Verification items for the finished model (mm, model axes). Face numbers are marked on the shaded views. Give positions to 0.01 mm unless a question says otherwise; leave off trailing zeros. Loops run counter-clockwise (first coordinate to the right, second up) from the corner with the lowest first, then second, coordinate; pieces in that order, holes last. Notation, with made-up numbers: (-22, 80.5) -> (7, 80.5) arc R17 cw to (7, 98.5) -> close; hole circle Ø2 at (-33, 51). An arc over 180 degrees is marked (long way). Answer in a Markdown table with one row per item. Add a question column.
Q1. Section check D-D on y = 13.5. Enter the section's corners in (x, z).
Q2. Section check B-B on x = 0. Enter the section's corners in (y, z).
Q3. Gauge pin test, flat ends, axial feed: P1, Ø0.5, axis at y = 11.5, z = 0.5, coming from the +X side; P2, Ø13, axis at x = 7.5, y = 2.5, coming from the +Z side; P3, Ø0.5, axis at y = 11.5, z = 0.5, coming from the -X side. Record the tip position at first contact, or that the pin passes through.
Q4. Section check A-A on y = 0. Enter the section's corners in (x, z).
Q5. Material ranges on probe 1 along X at (y, z) = (0, -0.2); probe 2 along X at (y, z) = (0, 0.2); probe 3 along Y at (x, z) = (0, -0.2), recorded low to high.
Q6. Release check for a two-part mould opening along Y. For the marked faces 1 and 2 record: pulls with the +Y half, pulls with the -Y half, needs draft (parallel to the pull), parting line crosses it, or undercut.
Q7. Section check C-C on z = 0.55. Enter the section's corners in (x, y).
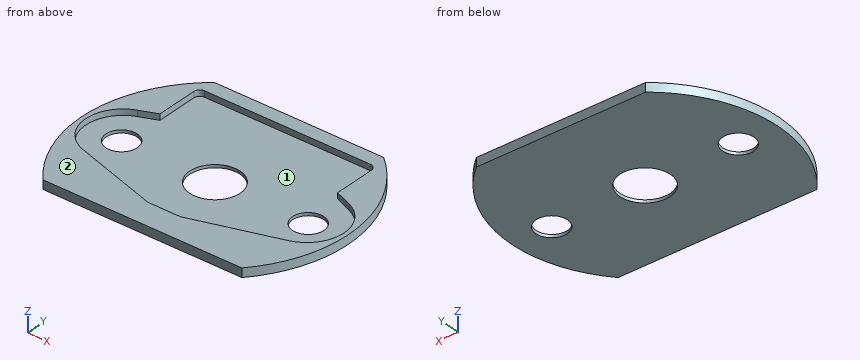
```python
from build123d import *

# Parameters (mm, degrees)
SKETCH_R        = 22.5
PAD_DEPTH       = 1
SKETCH001_R     = 22.5
PAD001_DEPTH    = 0.5
SKETCH002_R     = 4.25
SKETCH002_R_2   = 2.65
POCKET_DEPTH    = 1.501
FILLET_R        = 1
FILLET001_R     = 1
POCKET001_DEPTH = 5


with BuildPart() as part:
    # Sketch → Pad (new body)
    with BuildSketch(Plane.XY):
        Circle(SKETCH_R)
        with BuildLine():
            ThreePointArc((17.347253, -6.023093), (21.794374, -0.266197), (17.849197, 5.84562))
            Line((15, 6.990635), (17.849197, 5.84562))
            Line((15, 15), (15, 6.990635))
            Line((-15, 15), (15, 15))
            Line((-15, 15), (-15, 6.990635))
            Line((-17.849197, 5.84562), (-15, 6.990635))
            ThreePointArc((-17.849197, 5.84562), (-21.794374, -0.266197), (-17.347253, -6.023093))
            Line((-17.347253, -6.023093), (-2.75, -10.5))
            Line((-2.75, -10.5), (2.75, -10.5))
            Line((17.347253, -6.023093), (2.75, -10.5))
        make_face(mode=Mode.SUBTRACT)
    extrude(amount=PAD_DEPTH)

    # Sketch001 (on Face12 of Pad) → Pad001 (join)
    with BuildSketch(Plane(origin=(0, 0, 0), x_dir=(1, 0, 0), z_dir=(0, 0, -1))):
        Circle(SKETCH001_R)
    extrude(amount=PAD001_DEPTH)

    # Sketch002 (on Face4 of Pad001) → Pocket (cut, through all)
    with BuildSketch(Plane(origin=(0, 0, -0.5), x_dir=(1, 0, 0), z_dir=(0, 0, -1))):
        Circle(SKETCH002_R)
        with Locations((-15.75, 0)):
            Circle(SKETCH002_R_2)
        with Locations((15.75, 0)):
            Circle(SKETCH002_R_2)
    extrude(amount=-POCKET_DEPTH, mode=Mode.SUBTRACT)

    # Fillet
    fillet_edges = [part.edges().sort_by_distance(p)[0] for p in [
        (15, 15, 0.5),
        (-15, 15, 0.5),
    ]]
    fillet(fillet_edges, radius=FILLET_R)

    # Fillet001
    fillet001_edges = [part.edges().sort_by_distance(p)[0] for p in [
        (-2.75, -10.5, 0.5),
        (2.75, -10.5, 0.5),
    ]]
    fillet(fillet001_edges, radius=FILLET001_R)

    # Sketch003 (on Face1 of Fillet001) → Pocket001 (cut)
    with BuildSketch(Plane.XY.offset(1)):
        with BuildLine():
            Line((-14.299143, 17.371946), (14.299143, 17.371946))
            ThreePointArc((14.299143, 17.371946), (0, 22.5), (-14.299143, 17.371946))
        make_face()
        with BuildLine():
            Line((16.788655, -14.979688), (-16.788655, -14.979688))
            ThreePointArc((-16.788655, -14.979688), (0, -22.5), (16.788655, -14.979688))
        make_face()
    extrude(amount=-POCKET001_DEPTH, mode=Mode.SUBTRACT)


solid = part.part
```
Taken from the geometry:
| question | item | result |
|---|---|---|
| 1 | outline | (-18, -0.5) -> (18, -0.5) -> (18, 1) -> (15, 1) -> (15, 0) -> (-15, 0) -> (-15, 1) -> (-18, 1) -> close |
| 2 | outline | (-14.98, -0.5) -> (-4.25, -0.5) -> (-4.25, 0) -> (-10.5, 0) -> (-10.5, 1) -> (-14.98, 1) -> close; (4.25, -0.5) -> (17.37, -0.5) -> (17.37, 1) -> (15, 1) -> (15, 0) -> (4.25, 0) -> close |
| 3 | P1 | stops at x = 19.49 |
| 3 | P2 | stops at z = 0 |
| 3 | P3 | stops at x = -19.49 |
| 4 | outline | (-22.5, -0.5) -> (-18.4, -0.5) -> (-18.4, 0) -> (-21.8, 0) -> (-21.8, 1) -> (-22.5, 1) -> close; (-13.1, -0.5) -> (-4.25, -0.5) -> (-4.25, 0) -> (-13.1, 0) -> close; (4.25, -0.5) -> (13.1, -0.5) -> (13.1, 0) -> (4.25, 0) -> close; (18.4, -0.5) -> (22.5, -0.5) -> (22.5, 1) -> (21.8, 1) -> (21.8, 0) -> (18.4, 0) -> close |
| 5 | probe 1 | x = -22.5 to -18.4, -13.1 to -4.25, 4.25 to 13.1, 18.4 to 22.5 |
| 5 | probe 2 | x = -22.5 to -21.8, 21.8 to 22.5 |
| 5 | probe 3 | y = -14.98 to -4.25, 4.25 to 17.37 |
| 6 | face 1 | undercut |
| 6 | face 2 | needs draft |
| 7 | outline | (-16.79, -14.98) -> (16.79, -14.98) arc R22.5 ccw to (14.3, 17.37) -> (-14.3, 17.37) arc R22.5 ccw to start; hole (-17.85, 5.85) arc R6.3 ccw to (-17.35, -6.02) -> (-2.89, -10.46) arc R1 ccw to (-2.6, -10.5) -> (2.6, -10.5) arc R1 ccw to (2.89, -10.46) -> (17.35, -6.02) arc R6.3 ccw to (17.85, 5.85) -> (15, 6.99) -> (15, 14) arc R1 ccw to (14, 15) -> (-14, 15) arc R1 ccw to (-15, 14) -> (-15, 6.99) -> close |
